Verification items for the finished model (mm, model axes). A direction names the side the tool comes from. Round coordinates to 2 decimals unless told otherwise and drop trailing zeros. Loops run counter-clockwise (first coordinate to the right, second up) from the corner with the lowest first, then second, coordinate; pieces in that order, holes last. Notation, with made-up numbers: (0.25, -33.75) - (56.25, -33.75) arc R18 cw to (56.25, -5.75) - close; hole circle Ø6 at (26, 87). An arc over 180 degrees is marked (long way). Use a Markdown table: item, result. Add a question column.
```python
from build123d import *
from OCP.BRepFilletAPI import BRepFilletAPI_MakeFillet

# Parameters (mm, degrees)
SKETCH1_W                  = 8
SKETCH1_H                  = 52
BOSS_EXTRUDE1_DEPTH        = 52
BOSS_EXTRUDE2_DEPTH        = 7
SKETCH1_4_R                = 13
SKETCH1_4_R_2              = 8
BOSS_EXTRUDE3_DEPTH        = 27
FILLET1_R                  = 25
FILLET1_R_2                = 6
FILLET1_R_3                = 13
F_12_0MM_DOWEL_HOLE1_D     = 7
F_12_0MM_DOWEL_HOLE1_DEPTH = 30
F_12_0MM_DOWEL_HOLE1_TIP   = 2.103012167


with BuildPart() as part:
    # Sketch1 → Boss-Extrude1 (new body)
    with BuildSketch(Plane.XY):
        with Locations((-4, 0)):
            Rectangle(SKETCH1_W, SKETCH1_H)
    extrude(amount=BOSS_EXTRUDE1_DEPTH)

    # Sketch1<3> → Boss-Extrude2 (add)
    with BuildSketch(Plane.XY):
        with BuildLine():
            Line((42, 20), (0, 20))
            Line((0, 20), (0, 4))
            Line((0, 4), (29.630683123, 4))
            ThreePointArc((29.630683123, 4), (44.02470746, 12.841361287), (55, 0))
            ThreePointArc((55, 0), (44.02470746, -12.841361287), (29.630683123, -4))
            Line((29.630683123, -4), (0, -4))
            Line((0, -4), (0, -20))
            Line((0, -20), (42, -20))
            ThreePointArc((42, -20), (62, 0), (42, 20))
        make_face()
    extrude(amount=BOSS_EXTRUDE2_DEPTH)

    # Sketch1<4> → Boss-Extrude3 (add)
    # profile 1 of 2: a face of its own
    with BuildSketch(Plane.XY):
        with Locations((42, 0)):
            Circle(SKETCH1_4_R)
        with Locations((42, 0)):
            Circle(SKETCH1_4_R_2, mode=Mode.SUBTRACT)
    # profile 2 of 2: a face of its own
    with BuildSketch(Plane.XY):
        with BuildLine():
            Line((29.630683123, 4), (0, 4))
            Line((0, 4), (0, -4))
            Line((0, -4), (29.630683123, -4))
            ThreePointArc((29.630683123, -4), (29, 0), (29.630683123, 4))
        make_face()
    extrude(amount=BOSS_EXTRUDE3_DEPTH)

    # Fillet1
    fillet1_edges_1 = [part.edges().sort_by_distance(p)[0] for p in [
        (0, 0, 27),
    ]]
    fillet1_edges_2 = [part.edges().sort_by_distance(p)[0] for p in [
        (0, -20, 3.5),
        (0, 20, 3.5),
    ]]
    fillet1 = BRepFilletAPI_MakeFillet(part.part.solid().wrapped)
    for e in fillet1_edges_1:
        fillet1.Add(FILLET1_R - 0.0001, e.wrapped)
    for e in fillet1_edges_2:
        fillet1.Add(FILLET1_R_2 - 0.0001, e.wrapped)
    add(Compound.cast(fillet1.Shape()), mode=Mode.REPLACE)  # a hair under: the kernel refuses the full size
    fillet1_2_edges = [part.edges().sort_by_distance(p)[0] for p in [
        (-4, -26, 52),
        (-4, 26, 52),
    ]]
    fillet(fillet1_2_edges, radius=FILLET1_R_3)

    # Ø12.0mm Dowel Hole1
    with Locations(Plane(origin=(0, 16, 39), x_dir=(0, 1, 0), z_dir=(1, 0, 0))):
        with Locations((0, 0), (-32, 0)):
            Hole(F_12_0MM_DOWEL_HOLE1_D / 2, depth=F_12_0MM_DOWEL_HOLE1_DEPTH)
            with Locations((0, 0, -(F_12_0MM_DOWEL_HOLE1_DEPTH + F_12_0MM_DOWEL_HOLE1_TIP / 2))):  # 118° drill point
                Cone(0, F_12_0MM_DOWEL_HOLE1_D / 2, F_12_0MM_DOWEL_HOLE1_TIP, mode=Mode.SUBTRACT)


solid = part.part
```
Q1. Section check A-A on x = -3. Record the cut outline in (y, z).
Q2. Thickness scan on line 1 along Y through (x, z) = (42, 17); line 2 along Y through (x, z) = (-3, 36); line 3 along X through (y, z) = (-23, 13). Record the ranges inside material, lowest first.
Q3. Release check for a two-part mould opening along Z. For faces 5 (the face through (27, 0, 0)), 6 (the face through (-4.06, -15.54, 42.47)), 7 (the face through (62, 0, 3)) record: +Z half, -Z half, draft (parallel to the pull), parting line (faces both ways), or undercut.
Q4. Go/stop test with flat-tipped pins: pin 1 Ø8 at (x, y) = (32.5, -1.5) entering from -Z; pin 2 Ø5.5 at (x, z) = (23, 4.5) entering from +Y; pin 3 Ø1.5 at (y, z) = (-12, 21) entering from +X; pin 4 Ø1 at (x, z) = (11.5, 10.5) entering from +Y. Record where each tip stops, or that it passes through.
Q5. Section check B-B on z = 40. Record the cut outline in (x, y), plus the area to 3 significant figures.
Q6. Section check D-D on y = -16. Record the cut outline in (x, z), plus the area to 3 significant figures.
Q7. Section check C-C on z = 10. Record the cut outline in (x, y).
Q8. Set-up check for faces 1 (the face through (15, 4, 19)), 2 (the face through (24, -20, 3)), 3 (the face through (0, -6, 26)), 4 (the face through (36, 6, 27)): record each of +Z, -Z, +X, -X, +Y, -Y from which the full face is reachable in a straight line by a thin tool's end or side.
Determined:
| question | item | result |
|---|---|---|
| 1 | outline | (-26, 0) - (26, 0) - (26, 39) arc R13 ccw to (13, 52) - (-13, 52) arc R13 ccw to (-26, 39) - close; hole circle Ø7 at (-16, 39); hole circle Ø7 at (16, 39) |
| 2 | line 1 | y = -13 to -8, 8 to 13 |
| 2 | line 2 | y = -26 to -17.8, -14.2 to 14.2, 17.8 to 26 |
| 2 | line 3 | x = -8 to 0 |
| 3 | face 5 | -Z half |
| 3 | face 6 | undercut |
| 3 | face 7 | draft |
| 4 | pin 1 | stops at z = 0 |
| 4 | pin 2 | stops at y = 20 |
| 4 | pin 3 | stops at x = 48.51 |
| 4 | pin 4 | stops at y = 4 |
| 5 | outline | (-8, -25.96) - (0, -25.96) - (0, -19.35) - (-8, -19.35) - close; (-8, -12.65) - (0, -12.65) - (0, -4) - (3.07, -4) - (3.07, 4) - (0, 4) - (0, 12.65) - (-8, 12.65) - close; (-8, 19.35) - (0, 19.35) - (0, 25.96) - (-8, 25.96) - close |
| 5 | area | 333 mm² |
| 6 | outline | (-8, 0) - (54, 0) - (54, 7) - (0, 7) - (0, 35.5) - (-8, 35.5) - close; (-8, 42.5) - (0, 42.5) - (0, 51.65) - (-8, 51.65) - close |
| 6 | area | 735 mm² |
| 7 | outline | (-8, -26) - (0, -26) - (0, -4) - (29.63, -4) arc R13 ccw (long way) to (29.63, 4) - (0, 4) - (0, 26) - (-8, 26) - close; hole circle Ø16 at (42, 0) |
| 8 | face 1 | +Z, +Y |
| 8 | face 2 | +Z, -Z, +X, -Y |
| 8 | face 3 | +Z |
| 8 | face 4 | +Z, +X, +Y, -Y |
